Build history of the part. All positions in model axes, mm. A direction names the side the tool comes from. Coordinates: 2 decimals unless noted, no trailing zeros. Loops run counter-clockwise (first coordinate to the right, second up) from the corner with the lowest first, then second, coordinate; pieces in that order, holes last.
(1) Slice it at C-C (x = 41.5). Give the cut face in (y, z), and give its area (3 significant figures).
(2) Tool access for faces 1 (the face through (76.04, 9.44, 9.55)), 2 (the face through (69.035, 39, 3)), 3 (the face through (10.94, 30.54, 11.24)): list every direction of +Z, -Z, +X, -X, +Y, -Y with a clear straight run to the whole face (end or side of a thin tool).
(3) Slice it at A-A (y = 44). Give the cut face in (x, z) (3 decimals).
(4) Wall check: L1, parallel to Y at x = 63, z = 3.5; L2, parallel to X at y = 36.5, z = 7.5; L3, parallel to X at y = 10.5, z = 16.5. Give the ranges that are in metal, low to high.
(5) Two-plate mould, pull along Y, no slides. Class faces 4 (the face through (39.4, 25.3, 16.4)), 5 (the face through (72.94, 30.54, 11.24)), 6 (the face through (0, 25, 9)): pulls with the +Y half, pulls with the -Y half, needs draft (parallel to the pull), parting line crosses it, or undercut.
(6) Slice it at B-B (x = 71). Give the cut face in (y, z), and give its area (3 significant figures).
(7) Slice it at D-D (z = 2.5). Give the number of separate pieces and of enclosed holes in the cut face, and give its area (3 significant figures).
(8) Flat gauge pins, fed straight in: P1, Ø5, axis at y = 37.5, z = 2, coming from the -X side (3 decimals); P2, Ø5, axis at x = 61, y = 16, coming from the +Z side; P3, Ø1.5, axis at y = 12.5, z = 4.5, coming from the -X side. Where does each tip first touch, or does it go through?
from build123d import *

# Parameters (mm, degrees)
F1_DEPTH       = 80
F3_DEPTH       = 25
F6_D           = 5
F6_START       = 3.8023749
F6_CBORE_D     = 9
F6_CBORE_DEPTH = 11
F7_W           = 58.0699953184
F7_H           = 13
F8_DEPTH       = 6


with BuildPart() as f1:
    # F0 (on Right) → F1 (new body)
    with BuildSketch(Plane.YZ):
        Polygon((0, 25), (0, 0), (50, 0), (50, 8), align=None)
    extrude(amount=F1_DEPTH)

    # F2 (on face) → F3 (cut)
    with BuildSketch(Plane(origin=(0, 0, 0), x_dir=(1, 0, 0), z_dir=(0, 0, -1))):
        with BuildLine():
            Line((0.3183541251, -19.1510552385), (7.5, 0))
            Line((7.5, 0), (0, 0))
            Line((0, 0), (0, -20.9066724808))
            ThreePointArc((0, -20.9066724808), (0.0802322527, -20.0145484353), (0.3183541251, -19.1510552385))
        make_face()
        with BuildLine():
            ThreePointArc((0.3183541122, -30.8489442991), (0.0802322494, -29.9854511186), (0, -29.0933270912))
            Line((0, -29.0933270912), (0, -50))
            Line((0, -50), (7.5, -50))
            Line((7.5, -50), (0.3183541122, -30.8489442991))
        make_face()
        with BuildLine():
            Line((80, -50), (80, -29.0933270912))
            ThreePointArc((80, -29.0933270912), (79.9197677506, -29.9854511186), (79.6816458878, -30.8489442991))
            Line((79.6816458878, -30.8489442991), (72.5, -50))
            Line((72.5, -50), (80, -50))
        make_face()
        with BuildLine():
            Line((80, 0), (72.5, 0))
            Line((72.5, 0), (79.6816458749, -19.1510552385))
            ThreePointArc((79.6816458749, -19.1510552385), (79.9197677473, -20.0145484353), (80, -20.9066724808))
            Line((80, -20.9066724808), (80, 0))
        make_face()
    extrude(amount=-F3_DEPTH, mode=Mode.SUBTRACT)

    # F6 (through all)
    # its depths count from where the whole tool has entered the part; down to there all is cleared
    with Locations(Plane(origin=(0, 1.8249691595, 5.3675563516), x_dir=(1, 0, 0), z_dir=(0, -0.3219027332, -0.9467727448)).offset(-F6_START)):
        with Locations((71, -23.3579222113), (9, -23.3579222113)):
            CounterBoreHole(F6_D / 2, F6_CBORE_D / 2, F6_CBORE_DEPTH)

    # F7 (on face) → F8 (cut)
    with BuildSketch(Plane(origin=(0, 0, 0), x_dir=(1, 0, 0), z_dir=(0, 0, -1))):
        with Locations((40, -38.5)):
            Rectangle(F7_W, F7_H)
    extrude(amount=-F8_DEPTH, mode=Mode.SUBTRACT)


solid = f1.part
Response values:
1. outline: (0, 0) - (32, 0) - (32, 6) - (45, 6) - (45, 0) - (50, 0) - (50, 8) - (0, 25) - close
1. area: 747 mm2
2. face 1: +Z, -Z, +X, -Y
2. face 2: -Z
2. face 3: none
3. outline: (5.25, 0) - (10.965, 0) - (10.965, 6) - (69.035, 6) - (69.035, 0) - (74.75, 0) - (74.75, 10.04) - (5.25, 10.04) - close
4. L1: y = 0 to 32, 45 to 50
4. L2: x = 2.44 to 77.56
4. L3: x = 3.56 to 76.44
5. face 4: pulls with the +Y half
5. face 5: undercut
5. face 6: needs draft
6. outline: (0, 0) - (19.92, 0) - (24.44, 13.31) - (26.34, 12.67) - (27.37, 15.7) - (0, 25) - close; (29.42, 0) - (50, 0) - (50, 8) - (32.1, 14.09) - (31.07, 11.06) - (32.97, 10.41) - close
6. area: 696 mm2
7. separate pieces: 1
7. enclosed holes: 3
7. area: 2,810 mm2
8. P1: stops at x = 1.875
8. P2: stops at z = 20.41
8. P3: stops at x = 2.53
